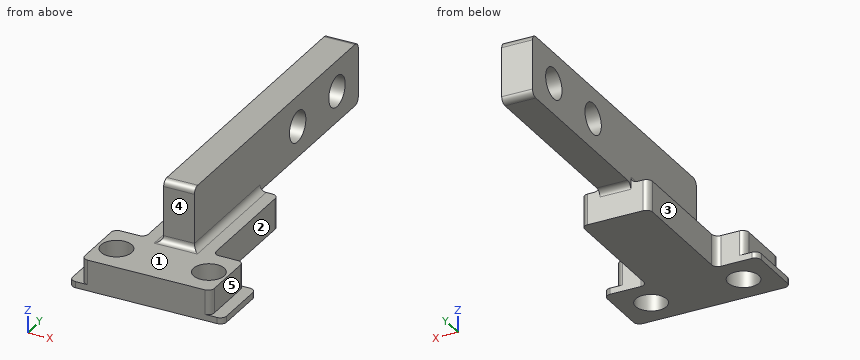
Autodesk Inventor part; units mm, degrees
ref_plane "YZ Plane" through (0, 0, 0) normal (1, 0, 0) x (0, 1, 0)
ref_plane "XZ Plane" through (0, 0, 0) normal (0, 1, 0) x (-1, 0, 0)
ref_plane "XY Plane" through (0, 0, 0) normal (0, 0, 1) x (1, 0, 0)
sketch "スケッチ6" plane through (0, 0, 0) normal (0, 0, 1) x (1, 0, 0)
  line L0 (0, 0) -> (25, 0)
  line L1 (25, 0) -> (25, 30)
  line L2 (25, 30) -> (0, 30)
  line L3 (0, 30) -> (0, 0)
  circle A0 centre (5, 5) radius 2.5
  circle A1 centre (20, 5) radius 2.5
  dimension "d39" = 5
  dimension "d40" = 5
  dimension "d41" = 5
  dimension "d42" = 5
  dimension "d43" = 15
  dimension "d44" = 5
  dimension "d45" = 5
  dimension "d46" = 30
extrude "押し出し4" add sketch "スケッチ6" along normal blind 5
sketch "スケッチ7" plane through (0, 0, 5) normal (0, 0, 1) x (1, 0, 0)
  line L0 (25, 30) -> (0, 30)
  line L1 (10, 30) -> (15, 30)
  line L2 (15, 30) -> (15, 10)
  line L3 (15, 10) -> (10, 10)
  line L4 (10, 10) -> (10, 30)
  line L5 (25, 0) -> (25, 30)
  line L6 (0, 30) -> (0, 0)
  line L7 (0, 0) -> (25, 0)
  line L8 (10, 30) -> (15, 30)
  line L9 (15, 30) -> (15, 60)
  line L10 (15, 60) -> (10, 60)
  line L11 (10, 60) -> (10, 30)
  dimension "d49" = 5
  dimension "d50" = 10
  dimension "d51" = 10
  dimension "d52" = 10
  dimension "d55" = 30
  dimension "d56" = 5
extrude "押し出し5" add sketch "スケッチ7" along normal blind 10 contours L2 L3 L4 L0 | L0 L11 L10 L9
sketch "スケッチ8" plane through (10, 30, 5) normal (-1, 0, 0) x (0, 0, 1)
  line L0 (10, 30) -> (10, -20)
  line L1 (0, 30) -> (10, 30)
  line L2 (0, -20) -> (10, -20)
  point P0 (-5, -30)
  point P1 (5, 11.5)
  point P2 (5, 23.5)
  dimension "d57" = 5
  dimension "d58" = 5
  dimension "d59" = 12
  dimension "d60" = 6.5
  dimension "d61" = 31.5
hole "穴3" at (10, 41.5, 10) at (10, 53.5, 10) direction (1, 0, 0) diameter 5 depth 8
sketch "スケッチ9" plane through (0, 0, 5) normal (0, 0, 1) x (1, 0, 0)
  line L0 (10, 30) -> (0, 30)
  line L1 (0, 30) -> (7, 30)
  line L2 (7, 30) -> (7, 10)
  line L3 (7, 10) -> (0, 10)
  line L4 (0, 10) -> (0, 30)
  line L5 (25, 0) -> (25, 30)
  line L6 (25, 30) -> (18, 30)
  line L7 (18, 30) -> (18, 10)
  line L8 (18, 10) -> (25, 10)
  line L9 (25, 10) -> (25, 30)
  point P0 (0, 0)
  point P1 (5, 30)
  point P2 (18, 20)
  point P3 (7, 20)
  dimension "d70" = 20
  dimension "d72" = 7
  dimension "d73" = 7
extrude "押し出し6" cut sketch "スケッチ9" against normal blind 10
fillet "フィレット4" radius 1 15 edges at (7, 30, 2.5) (12.5, 60, 5) (12.5, 60, 15) (12.5, 10, 15) (7, 10, 2.5) (0, 10, 2.5) (0, 0, 2.5) (18, 30, 2.5) (18, 10, 2.5) (25, 10, 2.5) (25, 0, 2.5) (10, 20, 5) (12.5, 30, 5) (15, 20, 5) (12.5, 10, 5)
sketch "スケッチ10" plane through (0, 0, 5) normal (0, 0, 1) x (1, 0, 0)
  line L0 (9, 30) -> (9, 9)
  line L1 (9, 30) -> (8, 30)
  arc A0 (8, 30) -> (7, 29) centre (8, 29) ccw
  line L2 (7, 29) -> (7, 11)
  arc A1 (6, 10) -> (7, 11) centre (6, 11) ccw
  line L3 (6, 10) -> (1, 10)
  arc A2 (1, 10) -> (0, 9) centre (1, 9) ccw
  line L4 (0, 9) -> (0, 1)
  arc A3 (0, 1) -> (1, 0) centre (1, 1) ccw
  line L5 (1, 0) -> (24, 0)
  arc A4 (24, 0) -> (25, 1) centre (24, 1) ccw
  line L6 (25, 1) -> (25, 9)
  arc A5 (25, 9) -> (24, 10) centre (24, 9) ccw
  line L7 (24, 10) -> (19, 10)
  arc A6 (18, 11) -> (19, 10) centre (19, 11) ccw
  line L8 (18, 11) -> (18, 29)
  arc A7 (18, 29) -> (17, 30) centre (17, 29) ccw
  line L9 (17, 30) -> (16, 30)
  line L10 (16, 9) -> (16, 30)
  line L11 (9, 9) -> (16, 9)
  circle A8 centre (5, 5) radius 2.5
  circle A9 centre (20, 5) radius 2.5
  line L12 (2, 8) -> (23, 8)
  line L13 (23, 8) -> (23, 2)
  line L14 (23, 2) -> (2, 2)
  line L15 (2, 2) -> (2, 8)
  line L16 (2, 10) -> (2, 0)
  line L17 (24, 10) -> (19, 10)
  line L18 (23, 10) -> (23, 0)
  point P0 (0, 0)
  point P1 (2, 2)
  point P2 (23, 2)
  dimension "d77" = 2
  dimension "d78" = 2
  dimension "d79" = 2
  dimension "d80" = 2
extrude "押し出し7" cut sketch "スケッチ10" against normal blind 4 contours L16 L15 L5 A3 L4 A2 L3 | L18 L7 A5 L6 A4 L5 L13
fillet "フィレット5" radius 1 4 edges at (23, 10, 3) (23, 0, 3) (2, 10, 3) (2, 0, 3)
equation "\"d42\" = d41"
equation "\"d45\" = d44"
equation "\"d73\" = d72"
properties part number "BP_BOX-Support-Bar-Connect1-Right" material "ABS プラスチック"
Could you check a few things on this model? Use its own coordinates, in mm. Face numbers are marked on the shaded views. A direction names the side the tool comes from. Coordinates: 2 decimals unless noted, no trailing zeros. Write each loop counter-clockwise with the first axis right and the second up, starting at its lowest first coordinate (ties: lowest second). Pieces come first, ordered by that corner, then holes. Notation, with made-up numbers: (-12, -1) -> (29, -1) arc R26 cw to (29, 27) -> close; hole circle Ø6 at (51.25, -19). An arc over 180 degrees is marked (long way). One line per question, with ' | ' between items. Start each with the question number.
1. Will these pins go through, and if not, where does the flat tip stop? P1, Ø0.9, axis at x = 23, y = 6, coming from the +Z side; P2, Ø6.5, axis at y = 41.5, z = 10, coming from the -X side; P3, Ø9, axis at y = 32, z = 7, coming from the -X side.
2. If we section it at A-A (y = 41.5): Please give me the cut outline in (x, z), and give its area (3 significant figures).
3. For the marked faces 1, 2, 3, 4 and 5, which set-ups out of +Z, -Z, +X, -X, +Y, -Y let a thin tool reach every point of the face, with its end or its side?
4. If we section it at D-D (x = 11): Please give me the cut outline in (y, z).
5. Please list where these lines run through material, in increasing order: line 1 along Y through (x, z) = (12.35, 10); line 2 along Z through (x, y) = (11.85, 53.5); line 3 along X through (y, z) = (31, 14).
6. If we section it at C-C (y = 5): Please give me the cut outline in (x, z).
7. If we section it at B-B (z = 10): Please give me the cut outline in (x, y), and give its area (3 significant figures).
Return value:
1) P1: stops at z = 5 | P2: stops at x = 10 | P3: stops at x = 7
2) outline: (10, 5) -> (15, 5) -> (15, 7.5) -> (10, 7.5) -> close; (10, 12.5) -> (15, 12.5) -> (15, 15) -> (10, 15) -> close | area: 25.0 mm²
3) face 1: +Z, -Y | face 2: +Z, -Z, +X, +Y | face 3: +Z, -Z, -X, +Y | face 4: +Z, +X, -X, -Y | face 5: +Z, +X, +Y, -Y
4) outline: (0, 0) -> (30, 0) -> (30, 4) arc R1 cw to (31, 5) -> (59, 5) arc R1 ccw to (60, 6) -> (60, 14) arc R1 ccw to (59, 15) -> (11, 15) arc R1 ccw to (10, 14) -> (10, 6) arc R1 cw to (9, 5) -> (0, 5) -> close; hole circle Ø5 at (41.5, 10); hole circle Ø5 at (53.5, 10)
5) line 1: y = 10 to 39, 44 to 51, 56 to 60 | line 2: z = 5 to 7.5, 12.5 to 15 | line 3: x = 10 to 15
6) outline: (0, 0) -> (2.5, 0) -> (2.5, 5) -> (2, 5) -> (2, 1) -> (0, 1) -> close; (7.5, 0) -> (17.5, 0) -> (17.5, 5) -> (7.5, 5) -> close; (22.5, 0) -> (25, 0) -> (25, 1) -> (23, 1) -> (23, 5) -> (22.5, 5) -> close
7) outline: (10, 10) -> (15, 10) -> (15, 39) -> (10, 39) -> close; (10, 44) -> (15, 44) -> (15, 51) -> (10, 51) -> close; (10, 56) -> (15, 56) -> (15, 60) -> (10, 60) -> close | area: 200 mm²
